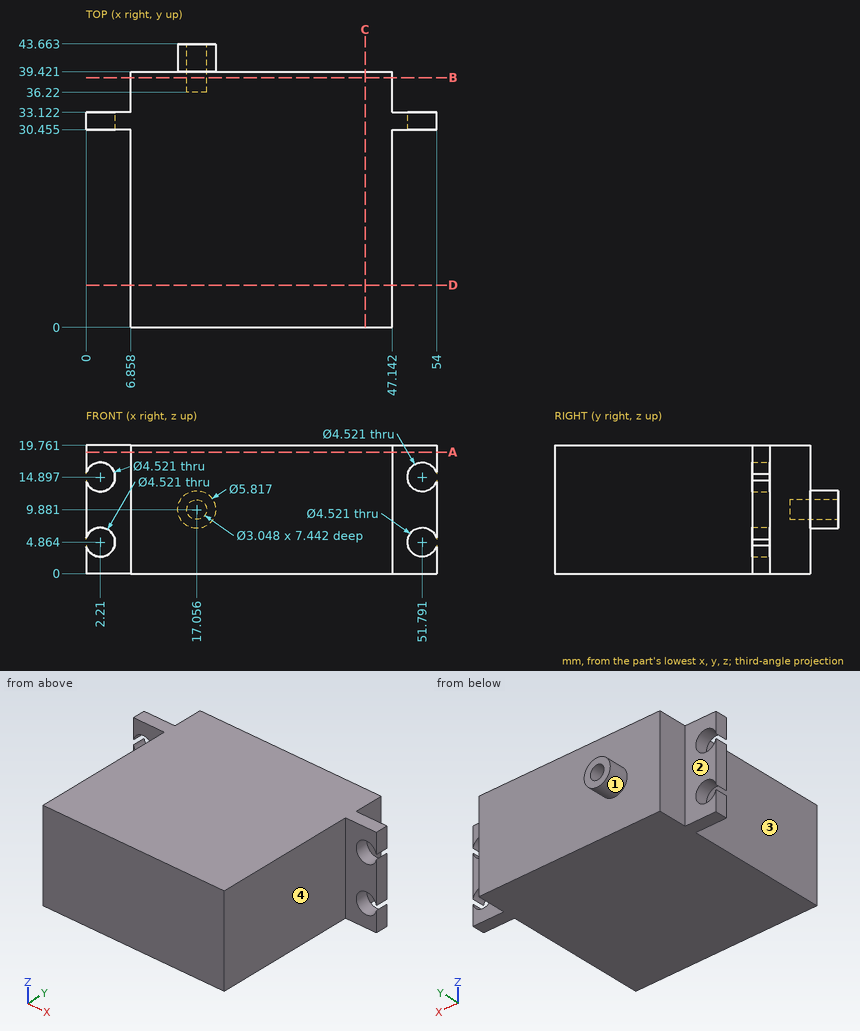
Answer from the drawing. Dimensions are ordinates in mm from the lowest x, y and z of the part. A direction names the side the tool comes from. Give positions to 0.01 mm unless a question says otherwise; leave off trailing zeros. Loops run counter-clockwise (first coordinate to the right, second up) from the corner with the lowest first, then second, coordinate; pieces in that order, holes last. Notation, with made-up numbers: (65.25, 19) -> (101.25, 19) arc R28 cw to (101.25, 46) -> close; hole circle Ø2 at (77.5, 5.5). An arc over 180 degrees is marked (long way). One line per question, with ' | ' between items. Start each with the question number.
1) For the marked faces 1, 2, 3 and 4, determine the directions among +Z, -Z, +X, -X, +Y, -Y from which every point of the face is accessible in a straight line to the end or side of a thin tool.
2) Section B-B, the plane y = 38.5 is taken. Determine the outline of the cut face in (x, z) (1 decimal), then the cut area to 3 significant figures.
3) Section D-D, the plane y = 6.5 is taken. Determine the outline of the cut face in (x, z), then the cut area to 3 significant figures.
4) Straight lines are drawn through the part: L1, parallel to X at y = 8, z = 11; L2, parallel to Y at x = 29, z = 4; L3, parallel to Y at x = 5, z = 4.75 (1 decimal). For each, find the intervals that lie inside material, in ascending order.
5) Section A-A, the plane z = 18.75 is taken. Determine the outline of the cut face in (x, y) (1 decimal), then the cut area to 3 significant figures.
6) Each of these flat-tipped pins is pushed along its axis until it touches: pin 1 (7.5 mm diameter, centred on x = 51, z = 10, fed in from -Y) (1 decimal); pin 2 (2 mm diameter, centred on x = 50.5, z = 13, fed in from +Y); pin 3 (1.9 mm diameter, centred on y = 35.5, z = 13, fed in from +X). Where does it stop, or does it pass through?
7) Section C-C, the plane x = 43 is taken. Determine the outline of the cut face in (y, z).
Resolved:
1) face 1: +Y | face 2: +Z, -Z, -X, +Y | face 3: +Z, -Z, -X, -Y | face 4: +Z, -Z, +X, -Y
2) outline: (6.9, 0) -> (47.1, 0) -> (47.1, 19.8) -> (6.9, 19.8) -> close; hole circle Ø3 at (17.1, 9.9) | area: 789 mm2
3) outline: (6.86, 0) -> (47.14, 0) -> (47.14, 19.76) -> (6.86, 19.76) -> close | area: 796 mm2
4) L1: 6.86 to 47.14 | L2: 0 to 39.42 | L3: 30.5 to 33.1
5) outline: (0, 30.5) -> (6.9, 30.5) -> (6.9, 0) -> (47.1, 0) -> (47.1, 30.5) -> (54, 30.5) -> (54, 33.1) -> (47.1, 33.1) -> (47.1, 39.4) -> (6.9, 39.4) -> (6.9, 33.1) -> (0, 33.1) -> close | area: 1,620 mm2
6) pin 1: y = 30.5 | pin 2: y = 33.12 | pin 3: x = 47.14
7) outline: (0, 0) -> (39.42, 0) -> (39.42, 19.76) -> (0, 19.76) -> close
